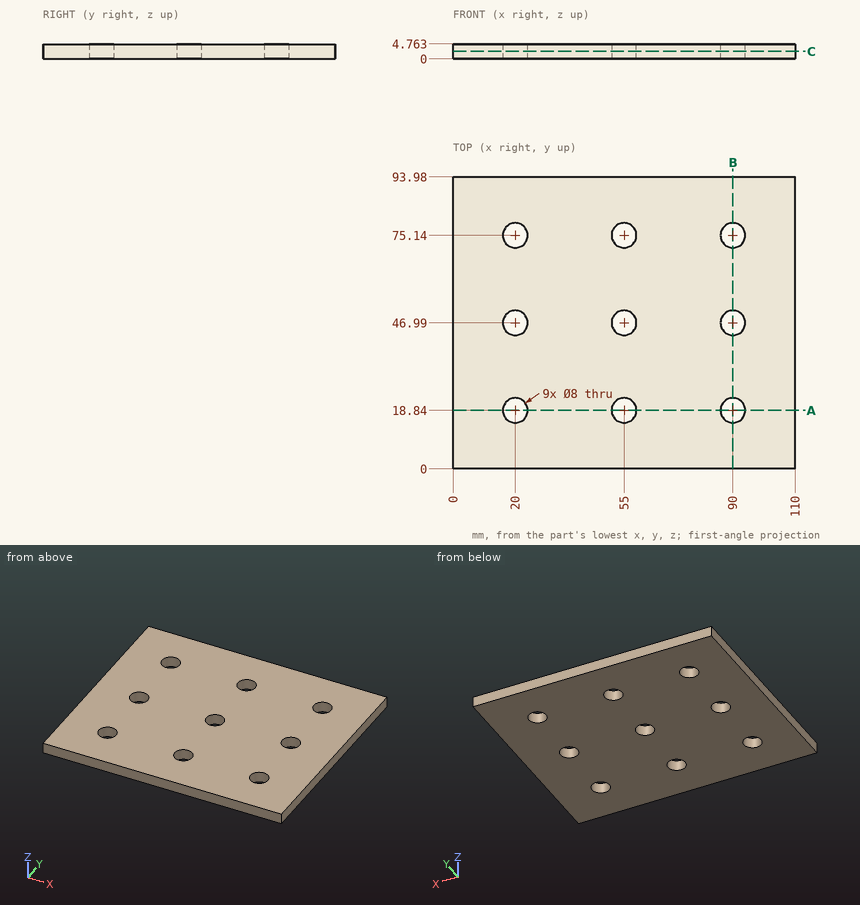
Geometry check sheet. Reference: drawing and pictorial views, mm from the part's lowest x, y, z. Coordinates: 2 decimals unless noted, no trailing zeros. Loops run counter-clockwise (first coordinate to the right, second up) from the corner with the lowest first, then second, coordinate; pieces in that order, holes last. Notation, with made-up numbers: (-15.5, 17) -> (13.5, 17) arc R18 cw to (13.5, 49) -> close; hole circle Ø11 at (30, 13.5). An arc over 180 degrees is marked (long way). Write item = value, one per line. Start each with the question number.
1. Section check B-B on x = 90. Record the cut outline in (y, z), then the cut area to 3 significant figures.
2. Material ranges on line 1 (Y direction, x = 90, z = 2.5); line 2 (X direction, y = 45, z = 3.8); line 3 (X direction, y = 21.5, z = 0.4) (1 decimal), recorded low to high.
3. Section check A-A on y = 18.84. Record the cut outline in (x, z).
4. Section check C-C on z = 2.4. Give the number of separate pieces and of enclosed holes in the cut face.
Responses:
q1.outline = (0, 0) -> (14.84, 0) -> (14.84, 4.76) -> (0, 4.76) -> close; (22.84, 0) -> (42.99, 0) -> (42.99, 4.76) -> (22.84, 4.76) -> close; (50.99, 0) -> (71.14, 0) -> (71.14, 4.76) -> (50.99, 4.76) -> close; (79.14, 0) -> (93.98, 0) -> (93.98, 4.76) -> (79.14, 4.76) -> close
q1.area = 333 mm2
q2.line_1 = 0 to 14.84, 22.84 to 42.99, 50.99 to 71.14, 79.14 to 93.98
q2.line_2 = 0 to 16.53, 23.47 to 51.53, 58.47 to 86.53, 93.47 to 110
q2.line_3 = 0 to 17, 23 to 52, 58 to 87, 93 to 110
q3.outline = (0, 0) -> (16, 0) -> (16, 4.76) -> (0, 4.76) -> close; (24, 0) -> (51, 0) -> (51, 4.76) -> (24, 4.76) -> close; (59, 0) -> (86, 0) -> (86, 4.76) -> (59, 4.76) -> close; (94, 0) -> (110, 0) -> (110, 4.76) -> (94, 4.76) -> close
q4.separate_pieces = 1
q4.enclosed_holes = 9
